Can you work these out from the drawing? Everything is in mm from the part's minimum corner. A direction names the side the tool comes from. Coordinates: 2 decimals unless noted, no trailing zeros. Order: outer loops, then holes, each group sorted by start corner. A loop starts at its lowest first (then second) coordinate and runs counter-clockwise, first axis right, second up. Notation, with made-up numbers: (-20.75, 15) -> (19.25, 15) arc R18 cw to (19.25, 24) -> close; hole circle Ø4 at (16.5, 29.5). An arc over 180 degrees is marked (long way). Write item = value, one per line. Start each with the question number.
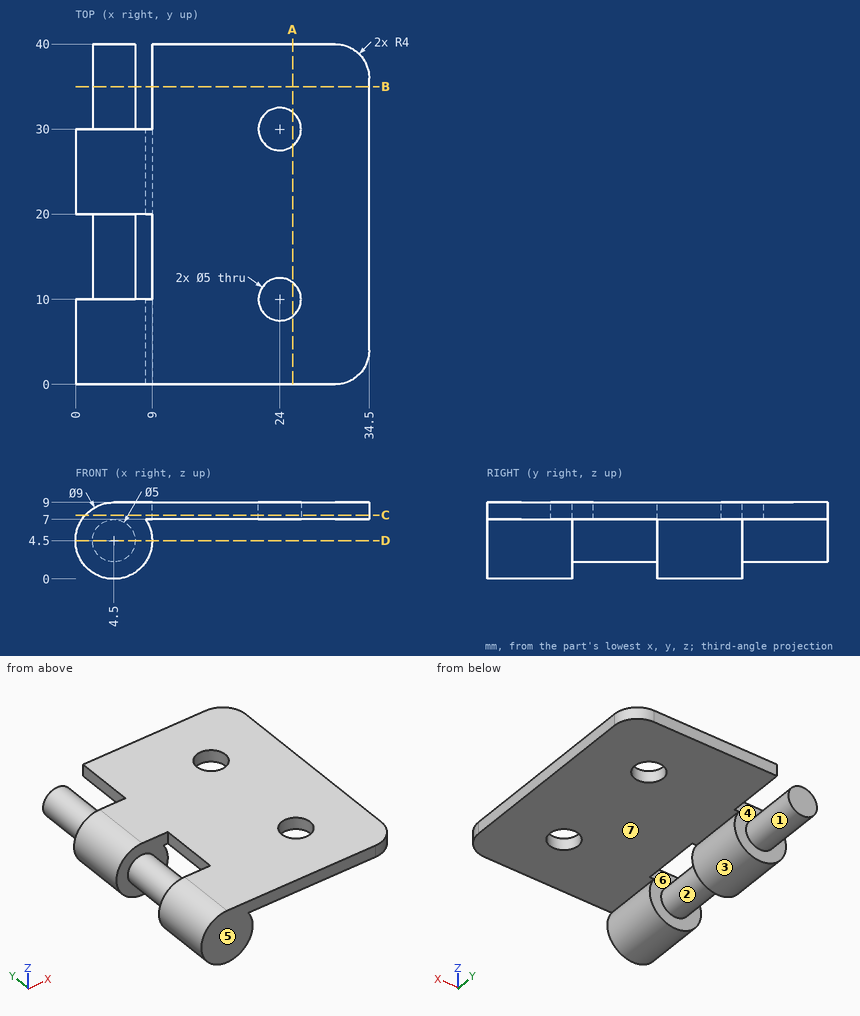
(1) If I drill on L1, parallel to Y at x = 24, z = 8.4; L2, parallel to Z at x = 16, y = 29; L3, parallel to X at y = 23, z = 3.25, over which ranges is the centre line in solid material (lowest first)? Write a range as from..to.
(2) Imagine slicing it at A-A (x = 25.5). Write out the boundary of the cut face in (y, z), plus the area to 3 significant figures.
(3) Imagine slicing it at C-C (z = 7.5). Write out the boundary of the cut face in (x, y).
(4) Imagine slicing it at B-B (y = 35). Write out the boundary of the cut face in (x, z), plus the area to 3 significant figures.
(5) Imagine slicing it at D-D (z = 4.5). Write out the boundary of the cut face in (x, y).
(6) For P1, Ø6.5, axis at x = 24, y = 10, coming from the -Z side; P2, Ø1, axis at y = 36, z = 8, coming from the -X side, each with a flat end and sliding along its axis, tell me the tip position at first contact or that it passes through.
(7) Thinking about a two-plate mould opening in Y: for the marked faces 4, 5, 6 and 7, which applies, +Y half, -Y half, draft (parallel to the pull), parting line (faces both ways), or undercut?
(8) For the marked faces 1, 2 and 3, which set-ups out of +Z, -Z, +X, -X, +Y, -Y let a thin tool reach every point of the face, with its end or its side?
Result set:
q1.L1 = 0..7.5, 12.5..27.5, 32.5..40
q1.L2 = 7..9
q1.L3 = 0.18..8.82
q2.outline = (0, 7) -> (8, 7) -> (8, 9) -> (0, 9) -> close; (12, 7) -> (28, 7) -> (28, 9) -> (12, 9) -> close; (32, 7) -> (40, 7) -> (40, 9) -> (32, 9) -> close
q2.area = 64.0 mm2
q3.outline = (1.15, 0) -> (30.5, 0) arc R4 ccw to (34.5, 4) -> (34.5, 36) arc R4 ccw to (30.5, 40) -> (9, 40) -> (9, 30) -> (1.15, 30) -> (1.15, 20) -> (9, 20) -> (9, 10) -> (1.15, 10) -> close; hole circle Ø5 at (24, 10); hole circle Ø5 at (24, 30)
q4.outline = circle Ø5 at (4.5, 4.5); (9, 7) -> (34.5, 7) -> (34.5, 9) -> (9, 9) -> close
q4.area = 70.6 mm2
q5.outline = (0, 0) -> (9, 0) -> (9, 10) -> (7, 10) -> (7, 20) -> (9, 20) -> (9, 30) -> (7, 30) -> (7, 40) -> (2, 40) -> (2, 30) -> (0, 30) -> (0, 20) -> (2, 20) -> (2, 10) -> (0, 10) -> close
q6.P1 = 7
q6.P2 = 9
q7.face_4 = +Y half
q7.face_5 = -Y half
q7.face_6 = undercut
q7.face_7 = draft
q8.face_1 = +Y
q8.face_2 = none
q8.face_3 = +Y, -Y
